The listing builds one solid part. Answer for the finished solid, in the listing's coordinates (mm). A direction names the side the tool comes from. Coordinates: 2 decimals unless noted, no trailing zeros. Order: outer loops, then holes, each group sorted by start corner. A loop starts at its lowest first (then second) coordinate and runs counter-clockwise, first axis right, second up. Notation, with made-up numbers: (39, 8.5) -> (92, 8.5) arc R9 cw to (92, 18.5) -> close; hole circle Ø8 at (84, -18). An arc over 180 degrees is marked (long way). Put each result on its own line as item: value. Start each with the question number.
```python
from build123d import *

# Parameters (mm, degrees)
SKETCH1_W           = 76
SKETCH1_H           = 10
BOSS_EXTRUDE1_DEPTH = 10
SKETCH2_W           = 9.046482833
SKETCH2_H           = 9.263922883
CUT_EXTRUDE1_DEPTH  = 77
SKETCH4_R           = 2.5
CUT_EXTRUDE2_DEPTH  = 76
SKETCH6_R           = 2.5
CUT_EXTRUDE3_DEPTH  = 76


with BuildPart() as part:
    # Sketch1 → Boss-Extrude1 (new body)
    with BuildSketch(Plane(origin=(0, 0, 0), x_dir=(1, 0, 0), z_dir=(0, 1, 0))):
        Rectangle(SKETCH1_W, SKETCH1_H)
    extrude(amount=BOSS_EXTRUDE1_DEPTH)

    # Sketch2 → Cut-Extrude1 (cut, through all)
    with BuildSketch(Plane.ZY.offset(38)):
        with Locations((-0.032492444, 5.042490422)):
            Rectangle(SKETCH2_W, SKETCH2_H)
    extrude(amount=-CUT_EXTRUDE1_DEPTH, mode=Mode.SUBTRACT)

    # Sketch4 → Cut-Extrude2 (cut)
    with BuildSketch(Plane.XY.offset(5)):
        with Locations((-28.218728934, 5)):
            Circle(SKETCH4_R)
    extrude(amount=-CUT_EXTRUDE2_DEPTH, mode=Mode.SUBTRACT)

    # Sketch6 → Cut-Extrude3 (cut)
    with BuildSketch(Plane(origin=(0, 10, 0), x_dir=(1, 0, 0), z_dir=(0, 1, 0))):
        with Locations((17, 0)):
            Circle(SKETCH6_R)
    extrude(amount=-CUT_EXTRUDE3_DEPTH, mode=Mode.SUBTRACT)


solid = part.part
```
(1) Find the intervals of material crossed by L1, parallel to X at y = 9.85, z = 0; L2, parallel to Y at x = -33.5, z = -3; L3, parallel to Z at x = -32.5, y = 2.25, in increasing order.
(2) The part is cut by section A-A on z = 0. Determine the outline of the cut face in (x, y).
(3) The part is cut by section B-B on x = -12. Determine the outline of the cut face in (y, z).
(4) For a pull along X with two mould halves and no side action, classify faces 3 (the flat face through (-38, 5, 4.8)), 4 (the flat face through (38, 5, 4.8)), 5 (the cylindrical face through (14.5, 0.2, -0.1)), 6 (the flat face through (-1, 5, 4.491)) as released by +X, released by -X, zero draft, split by the parting line, or undercut.
(5) This flat-tipped pin is pushed along its axis until it touches: P1, Ø1.5, axis at y = 7, z = 2, coming from the -X side. Where does it stop, or does it pass through?
(6) The part is cut by section C-C on x = -29. Determine the outline of the cut face in (y, z), plus the area to 3 significant figures.
(7) A tool of negligible diameter and unlimited length cuts with its end or side. For faces 1 (the cylindrical face through (-30.06, 6.69, 4.75)), 2 (the flat face through (-1, 0.411, 0)), from which of +Z, -Z, +X, -X, +Y, -Y can it reach the whole face along a straight path? Write none if from no direction.
Worked out:
1. L1: -38 to 14.5, 19.5 to 38
1. L2: 0 to 0.41, 9.67 to 10
1. L3: -5 to -4.56, 4.49 to 5
2. outline: (-38, 0) -> (14.5, 0) -> (14.5, 0.41) -> (-38, 0.41) -> close; (-38, 9.67) -> (14.5, 9.67) -> (14.5, 10) -> (-38, 10) -> close; (19.5, 0) -> (38, 0) -> (38, 0.41) -> (19.5, 0.41) -> close; (19.5, 9.67) -> (38, 9.67) -> (38, 10) -> (19.5, 10) -> close
3. outline: (0, -5) -> (10, -5) -> (10, 5) -> (0, 5) -> close; hole (0.41, -4.56) -> (9.67, -4.56) -> (9.67, 4.49) -> (0.41, 4.49) -> close
4. face 3: released by -X
4. face 4: released by +X
4. face 5: undercut
4. face 6: zero draft
5. P1: through
6. outline: (0, -5) -> (2.63, -5) -> (2.63, -4.56) -> (0.41, -4.56) -> (0.41, 4.49) -> (2.63, 4.49) -> (2.63, 5) -> (0, 5) -> close; (7.37, -5) -> (10, -5) -> (10, 5) -> (7.37, 5) -> (7.37, 4.49) -> (9.67, 4.49) -> (9.67, -4.56) -> (7.37, -4.56) -> close
6. area: 11.7 mm2
7. face 1: +Z, -Z
7. face 2: +X, -X
